Build history of the part. All positions in model axes, mm. Face numbers are marked on the shaded views. A direction names the side the tool comes from. Coordinates: 2 decimals unless noted, no trailing zeros. Write each loop counter-clockwise with the first axis right and the second up, starting at its lowest first coordinate (ties: lowest second). Pieces come first, ordered by that corner, then holes.
```python
from build123d import *

# Parameters (mm, degrees)
ESQUISSE1_R             = 5
BOSS_EXTRU_2_DEPTH      = 70
ESQUISSE2_R             = 3.5
BOSS_EXTRU_3_DEPTH      = 12
ESQUISSE4_R             = 15
BOSS_EXTRU_5_DEPTH      = 5
ESQUISSE5_R             = 3.5
BOSS_EXTRU_6_DEPTH      = 12
ENL_V_MAT_EXTRU_1_DEPTH = 12
ESQUISSE7_R             = 5
ENL_V_MAT_EXTRU_2_DEPTH = 47
ESQUISSE8_W             = 14
ESQUISSE8_H             = 14
BOSS_EXTRU_7_DEPTH      = 5
ESQUISSE9_W             = 14
ESQUISSE9_H             = 14
ESQUISSE9_W_2           = 8
ESQUISSE9_H_2           = 8
BOSS_EXTRU_8_DEPTH      = 4.5
ESQUISSE10_W            = 8
ESQUISSE10_H            = 8
ENL_V_MAT_EXTRU_3_DEPTH = 3.5
ESQUISSE12_W            = 14
ESQUISSE12_H            = 14
ESQUISSE12_W_2          = 8
ESQUISSE12_H_2          = 8
BOSS_EXTRU_9_DEPTH      = 4
ESQUISSE14_W            = 8
ESQUISSE14_H            = 8
ENL_V_MAT_EXTRU_4_DEPTH = 2
ESQUISSE15_R            = 2.5
ENL_V_MAT_EXTRU_5_DEPTH = 2
ESQUISSE16_W            = 8
ESQUISSE16_H            = 8
ENL_V_MAT_EXTRU_6_DEPTH = 2
ESQUISSE17_R            = 2.5
ENL_V_MAT_EXTRU_7_DEPTH = 2
ESQUISSE18_R            = 4
BOSS_EXTRU_10_DEPTH     = 12


with BuildPart() as part:
    # Esquisse1 → Boss.-Extru.2 (new body)
    with BuildSketch(Plane.XY):
        Circle(ESQUISSE1_R)
    extrude(amount=BOSS_EXTRU_2_DEPTH)

    # Esquisse2 → Boss.-Extru.3 (add)
    with BuildSketch(Plane(origin=(0, 0, 0), x_dir=(-1, 0, 0), z_dir=(0, 0, -1))):
        Circle(ESQUISSE2_R)
    extrude(amount=BOSS_EXTRU_3_DEPTH)

    # Esquisse4 → Boss.-Extru.5 (add)
    with BuildSketch(Plane.XY.offset(70)):
        Circle(ESQUISSE4_R)
    extrude(amount=-BOSS_EXTRU_5_DEPTH)

    # Esquisse5 → Boss.-Extru.6 (add)
    with BuildSketch(Plane.XY.offset(70)):
        Circle(ESQUISSE5_R)
    extrude(amount=BOSS_EXTRU_6_DEPTH)

    # Esquisse6 → Enlèv. mat.-Extru.1 (cut)
    with BuildSketch(Plane.XY.offset(70)):
        with BuildLine():
            Line((-6.262893089, 8.172072336), (-7.499435292, 12.990707074))
            ThreePointArc((-7.499435292, 12.990707074), (-9.123657799, 11.90625333), (-10.593218546, 10.619968024))
            Line((-10.593218546, 10.619968024), (-6.262893089, 8.172072336))
        make_face()
        with BuildLine():
            Line((-8.152402023, 6.270263162), (-10.606442664, 10.606760769))
            ThreePointArc((-10.606442664, 10.606760769), (-11.894621233, 9.138817524), (-12.981158937, 7.515950549))
            Line((-12.981158937, 7.515950549), (-8.152402023, 6.270263162))
        make_face()
        with BuildLine():
            Line((-9.499942261, 3.951679007), (-12.981158937, 7.515950549))
            ThreePointArc((-12.981158937, 7.515950549), (-13.849269023, 5.761748652), (-14.481582106, 3.909447494))
            Line((-14.481582106, 3.909447494), (-9.499942261, 3.951679007))
        make_face()
        with BuildLine():
            Line((-10.188028074, 1.356459322), (-14.486441985, 3.891400598))
            ThreePointArc((-14.486441985, 3.891400598), (-14.869805294, 1.972027008), (-14.999987869, 0.0190767))
            Line((-14.999987869, 0.0190767), (-10.188028074, 1.356459322))
        make_face()
        with BuildLine():
            ThreePointArc((-14.999987869, -0.0190767), (-14.869805294, -1.972027008), (-14.486441985, -3.891400598))
            Line((-14.486441985, -3.891400598), (-10.188028074, -1.356459322))
            Line((-10.188028074, -1.356459322), (-14.999987869, -0.0190767))
        make_face()
        with BuildLine():
            Line((-9.499942261, -3.951679007), (-14.481582106, -3.909447494))
            ThreePointArc((-14.481582106, -3.909447494), (-13.849269023, -5.761748652), (-12.981158937, -7.515950549))
            Line((-12.981158937, -7.515950549), (-9.499942261, -3.951679007))
        make_face()
        with BuildLine():
            Line((-8.152402023, -6.270263162), (-12.981158937, -7.515950549))
            ThreePointArc((-12.981158937, -7.515950549), (-11.894621233, -9.138817524), (-10.606442664, -10.606760769))
            Line((-10.606442664, -10.606760769), (-8.152402023, -6.270263162))
        make_face()
        with BuildLine():
            Line((-6.262893089, -8.172072336), (-10.593218546, -10.619968024))
            ThreePointArc((-10.593218546, -10.619968024), (-9.123657799, -11.90625333), (-7.499435292, -12.990707074))
            Line((-7.499435292, -12.990707074), (-6.262893089, -8.172072336))
        make_face()
        with BuildLine():
            Line((-3.939593974, -9.504960245), (-7.499435292, -12.990707074))
            ThreePointArc((-7.499435292, -12.990707074), (-5.744130769, -13.8565855), (-3.891026946, -14.486542352))
            Line((-3.891026946, -14.486542352), (-3.939593974, -9.504960245))
        make_face()
        with BuildLine():
            Line((-1.343501295, -10.189744953), (-3.872973884, -14.491379275))
            ThreePointArc((-3.872973884, -14.491379275), (-1.953114292, -14.872301253), (0, -15))
            Line((0, -15), (-1.343501295, -10.189744953))
        make_face()
        with BuildLine():
            ThreePointArc((0, -15), (1.953114292, -14.872301253), (3.872973884, -14.491379275))
            Line((3.872973884, -14.491379275), (1.343501295, -10.189744953))
            Line((1.343501295, -10.189744953), (0, -15))
        make_face()
        with BuildLine():
            ThreePointArc((3.891026946, -14.486542352), (5.744130769, -13.8565855), (7.499435292, -12.990707074))
            Line((7.499435292, -12.990707074), (3.939593974, -9.504960245))
            Line((3.939593974, -9.504960245), (3.891026946, -14.486542352))
        make_face()
        with BuildLine():
            ThreePointArc((7.499435292, -12.990707074), (9.123657799, -11.90625333), (10.593218546, -10.619968024))
            Line((10.593218546, -10.619968024), (6.262893089, -8.172072336))
            Line((6.262893089, -8.172072336), (7.499435292, -12.990707074))
        make_face()
        with BuildLine():
            ThreePointArc((10.606442664, -10.606760769), (11.894621233, -9.138817524), (12.981158937, -7.515950549))
            Line((12.981158937, -7.515950549), (8.152402023, -6.270263162))
            Line((8.152402023, -6.270263162), (10.606442664, -10.606760769))
        make_face()
        with BuildLine():
            ThreePointArc((12.981158937, -7.515950549), (13.849269023, -5.761748652), (14.481582106, -3.909447494))
            Line((14.481582106, -3.909447494), (9.499942261, -3.951679007))
            Line((9.499942261, -3.951679007), (12.981158937, -7.515950549))
        make_face()
        with BuildLine():
            ThreePointArc((15, 0), (14.999996967, 0.009538352), (14.999987869, 0.0190767))
            Line((14.999987869, 0.0190767), (10.159352957, -1.339548494))
            Line((10.159352957, -1.339548494), (14.486441985, -3.891400598))
            ThreePointArc((14.486441985, -3.891400598), (14.87105628, -1.962571047), (15, 0))
        make_face()
        with BuildLine():
            ThreePointArc((14.999987869, 0.0190767), (14.869805294, 1.972027008), (14.486441985, 3.891400598))
            Line((14.486441985, 3.891400598), (10.188028074, 1.356459322))
            Line((10.188028074, 1.356459322), (14.999987869, 0.0190767))
        make_face()
        with BuildLine():
            ThreePointArc((14.481582106, 3.909447494), (13.849269023, 5.761748652), (12.981158937, 7.515950549))
            Line((12.981158937, 7.515950549), (9.499942261, 3.951679007))
            Line((9.499942261, 3.951679007), (14.481582106, 3.909447494))
        make_face()
        with BuildLine():
            ThreePointArc((12.981158937, 7.515950549), (11.894621233, 9.138817524), (10.606442664, 10.606760769))
            Line((10.606442664, 10.606760769), (8.152402023, 6.270263162))
            Line((8.152402023, 6.270263162), (12.981158937, 7.515950549))
        make_face()
        with BuildLine():
            ThreePointArc((10.593218546, 10.619968024), (9.123657799, 11.90625333), (7.499435292, 12.990707074))
            Line((7.499435292, 12.990707074), (6.262893089, 8.172072336))
            Line((6.262893089, 8.172072336), (10.593218546, 10.619968024))
        make_face()
        with BuildLine():
            ThreePointArc((7.499435292, 12.990707074), (5.744130769, 13.8565855), (3.891026946, 14.486542352))
            Line((3.891026946, 14.486542352), (3.939593974, 9.504960245))
            Line((3.939593974, 9.504960245), (7.499435292, 12.990707074))
        make_face()
        with BuildLine():
            ThreePointArc((3.872973884, 14.491379275), (1.953114292, 14.872301253), (0, 15))
            Line((0, 15), (1.343501295, 10.189744953))
            Line((1.343501295, 10.189744953), (3.872973884, 14.491379275))
        make_face()
        with BuildLine():
            Line((-1.343501295, 10.189744953), (0, 15))
            ThreePointArc((0, 15), (-1.953114292, 14.872301253), (-3.872973884, 14.491379275))
            Line((-3.872973884, 14.491379275), (-1.343501295, 10.189744953))
        make_face()
        with BuildLine():
            Line((-3.939593974, 9.504960245), (-3.891026946, 14.486542352))
            ThreePointArc((-3.891026946, 14.486542352), (-5.744130769, 13.8565855), (-7.499435292, 12.990707074))
            Line((-7.499435292, 12.990707074), (-3.939593974, 9.504960245))
        make_face()
    extrude(amount=-ENL_V_MAT_EXTRU_1_DEPTH, mode=Mode.SUBTRACT)

    # Esquisse7 → Enlèv. mat.-Extru.2 (cut)
    with BuildSketch(Plane(origin=(0, 0, -12), x_dir=(-1, 0, 0), z_dir=(0, 0, -1))):
        Circle(ESQUISSE7_R)
    extrude(amount=-ENL_V_MAT_EXTRU_2_DEPTH, mode=Mode.SUBTRACT)

    # Esquisse8 → Boss.-Extru.7 (add)
    with BuildSketch(Plane(origin=(0, 0, 35), x_dir=(-1, 0, 0), z_dir=(0, 0, -1))):
        Rectangle(ESQUISSE8_W, ESQUISSE8_H)
    extrude(amount=-BOSS_EXTRU_7_DEPTH)

    # Esquisse9 → Boss.-Extru.8 (add)
    with BuildSketch(Plane(origin=(0, 0, 35), x_dir=(-1, 0, 0), z_dir=(0, 0, -1))):
        Rectangle(ESQUISSE9_W, ESQUISSE9_H)
        Rectangle(ESQUISSE9_W_2, ESQUISSE9_H_2, mode=Mode.SUBTRACT)
    extrude(amount=BOSS_EXTRU_8_DEPTH)

    # Esquisse10 → Enlèv. mat.-Extru.3 (cut)
    with BuildSketch(Plane(origin=(0, 0, 35), x_dir=(-1, 0, 0), z_dir=(0, 0, -1))):
        Rectangle(ESQUISSE10_W, ESQUISSE10_H)
    extrude(amount=-ENL_V_MAT_EXTRU_3_DEPTH, mode=Mode.SUBTRACT)

    # Esquisse12 → Boss.-Extru.9 (add)
    with BuildSketch(Plane(origin=(0, 0, 30.5), x_dir=(-1, 0, 0), z_dir=(0, 0, -1))):
        Rectangle(ESQUISSE12_W, ESQUISSE12_H)
        Rectangle(ESQUISSE12_W_2, ESQUISSE12_H_2, mode=Mode.SUBTRACT)
    extrude(amount=BOSS_EXTRU_9_DEPTH)

    # Esquisse14 → Enlèv. mat.-Extru.4 (cut)
    with BuildSketch(Plane.ZY.offset(7)):
        with Locations((33, 0)):
            Rectangle(ESQUISSE14_W, ESQUISSE14_H)
    extrude(amount=-ENL_V_MAT_EXTRU_4_DEPTH, mode=Mode.SUBTRACT)

    # Esquisse15 → Enlèv. mat.-Extru.5 (cut)
    with BuildSketch(Plane.ZY.offset(5)):
        with Locations((33, 0)):
            Circle(ESQUISSE15_R)
    extrude(amount=-ENL_V_MAT_EXTRU_5_DEPTH, mode=Mode.SUBTRACT)

    # Esquisse16 → Enlèv. mat.-Extru.6 (cut)
    with BuildSketch(Plane(origin=(7, 0, 0), x_dir=(0, 0, -1), z_dir=(1, 0, 0))):
        with Locations((-33, 0)):
            Rectangle(ESQUISSE16_W, ESQUISSE16_H)
    extrude(amount=-ENL_V_MAT_EXTRU_6_DEPTH, mode=Mode.SUBTRACT)

    # Esquisse17 → Enlèv. mat.-Extru.7 (cut)
    with BuildSketch(Plane(origin=(5, 0, 0), x_dir=(0, 0, -1), z_dir=(1, 0, 0))):
        with Locations((-33, 0)):
            Circle(ESQUISSE17_R)
    extrude(amount=-ENL_V_MAT_EXTRU_7_DEPTH, mode=Mode.SUBTRACT)

    # Esquisse18 → Boss.-Extru.10 (add)
    with BuildSketch(Plane.XY.offset(82)):
        Circle(ESQUISSE18_R)
    extrude(amount=-BOSS_EXTRU_10_DEPTH)


solid = part.part
```
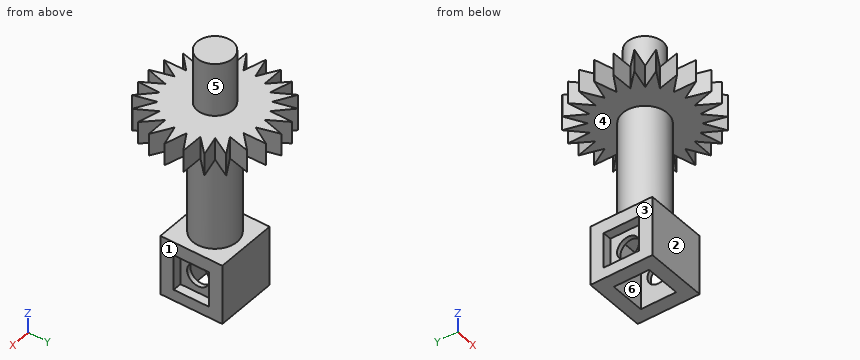
1. 3-axis set-ups, long thin cutter, end or side, ignore diameter. For the marked faces 1, 2 and 3: which of +Z, -Z, +X, -X, +Y, -Y reach the whole face in a straight line?
Computed values:
face 1: -Z, +X, +Y, -Y
face 2: -Z, +X, -X, -Y
face 3: -Z, -X, +Y, -Y
2. Mould opens along Y. For the marked faces 4, 5 and 6 say: +Y half, -Y half, draft (parallel to the pull), parting line (faces both ways), or undercut.
Computed values:
face 4: draft
face 5: parting line
face 6: undercut
3. Saw through at C-C on z = 55.5. List the corners of the cut face in (x, y), plus the area to 3 significant figures.
Computed values:
outline: circle Ø10 at (0, 0)
area: 78.5 mm2
4. Probe line 1 along Y through (x, z) = (4.3, 33); line 2 along Z through (x, y) = (-2.5, 6.25); line 3 along X through (y, z) = (-4.75, 37). List the from-to ranges inside material, lowest first.
Computed values:
line 1: y = -7 to -2.5, 2.5 to 7
line 2: z = 26.5 to 40, 65 to 70
line 3: x = -7 to 7
5. Flat gauge pins, fed straight in: pin 1 (1 mm diameter, centred on y = 4.5, z = 70, fed in from +X); pin 2 (6.5 mm diameter, centred on y = 0, z = 33, fed in from -X); pin 3 (2 mm diameter, centred on x = -6.5, y = 1.5, fed in from +Z); pin 4 (4.5 mm diameter, centred on y = 0, z = 33, fed in from +X). Where does each tip first touch, or does it go through?
Computed values:
pin 1: stops at x = 10.52
pin 2: stops at x = -5
pin 3: stops at z = 70
pin 4: passes through
6. Saw through at A-A on z = 33. List the corners of the cut face in (x, y).
Computed values:
outline: (-7, -7) - (7, -7) - (7, -4) - (5, -4) - (5, -2.5) - (4, -2.5) - (4, -4) - (-4, -4) - (-4, -2.5) - (-5, -2.5) - (-5, -4) - (-7, -4) - close; (-7, 4) - (-5, 4) - (-5, 2.5) - (-4, 2.5) - (-4, 4) - (4, 4) - (4, 2.5) - (5, 2.5) - (5, 4) - (7, 4) - (7, 7) - (-7, 7) - close
7. Saw through at B-B on z = 73.5. List the corners of the cut face in (x, y).
Computed values:
outline: circle Ø8 at (0, 0)
